Check sheet for the modelled part. Datum: model origin and axes. Units: mm. A direction names the side the tool comes from. Give positions to 0.01 mm unless a question says otherwise; leave off trailing zeros. Write each loop counter-clockwise with the first axis right and the second up, starting at its lowest first coordinate (ties: lowest second). Pieces come first, ordered by that corner, then holes. Notation, with made-up numbers: M 72,-26.75 L 130,-26.75 A13 ccw 130,-5.75 Z; hole C 59.5,-16.5 d10. An arc over 180 degrees is marked long. Write each question's results on one line, items separated by ' | '. Start each with the question number.
from build123d import *

# Parameters (mm, degrees)
SKETCH1_R           = 1.75
BOSS_EXTRUDE1_DEPTH = 10
BOSS_EXTRUDE2_DEPTH = 105
RIB1_REACH          = 140.024
SKETCH3_WALL_W      = 372.917163166
SKETCH3_WALL_H      = 6
FILLET1_R           = 2
FILLET2_R           = 4
SKETCH4_W           = 4
SKETCH4_H           = 13.56
CUT_EXTRUDE1_DEPTH  = 8


with BuildPart() as part:
    # Sketch1 → Boss-Extrude1 (new body)
    with BuildSketch(Plane.XY):
        Polygon((-45.99, 7.5), (-45.99, -7.5), (-17.99, -7.5), (-17.99, -53.64), (46, -53.64), (46, -38.64), (31.39, -38.64), (31.39, 7.5), align=None)
        Circle(SKETCH1_R, mode=Mode.SUBTRACT)
        with Locations((25.39, 0)):
            Circle(SKETCH1_R, mode=Mode.SUBTRACT)
        with Locations((-39.99, 0)):
            Circle(SKETCH1_R, mode=Mode.SUBTRACT)
        with Locations((40, -46.14)):
            Circle(SKETCH1_R, mode=Mode.SUBTRACT)
    extrude(amount=BOSS_EXTRUDE1_DEPTH)

    # Sketch2 → Boss-Extrude2 (add)
    with BuildSketch(Plane.XY.offset(10)):
        Polygon((-13.3, -5), (-3.3, -5), (-3.3, -18.56), (-13.3, -18.56), (-13.3, -12.56), (-8.3, -12.56), (-8.3, -10), (-13.3, -10), align=None)
    extrude(amount=BOSS_EXTRUDE2_DEPTH)

    # Sketch3 wall → Rib1 (add, up to next)
    with BuildSketch(Plane(origin=(-8.3, -33.56, 55), x_dir=(0, 0.316227766017, 0.948683298051), z_dir=(0, -0.948683298051, 0.316227766017)), mode=Mode.PRIVATE) as rib1_sk1:
        Rectangle(SKETCH3_WALL_W, SKETCH3_WALL_H)
    rib1_tool1 = extrude(rib1_sk1.sketch, amount=-RIB1_REACH, mode=Mode.PRIVATE) - part.part
    add(rib1_tool1.solids().sort_by_distance((-8.3, -33.56, 55))[0])

    # Fillet1
    fillet1_edges = [part.edges().sort_by_distance(p)[0] for p in [
        (-13.3, -7.5, 10),
        (-13.3, -15.56, 10),
        (-12.3, -18.56, 10),
        (-11.3, -33.56, 10),
        (-3.3, -11.78, 10),
        (-4.3, -18.56, 10),
        (-5.3, -33.56, 10),
    ]]
    fillet(fillet1_edges, radius=FILLET1_R)

    # Fillet2
    fillet2_edges = [part.edges().sort_by_distance(p)[0] for p in [
        (31.39, -38.64, 5),
        (-17.99, -53.64, 5),
        (-17.99, -7.5, 5),
    ]]
    fillet(fillet2_edges, radius=FILLET2_R)

    # Sketch4 → Cut-Extrude1 (cut)
    with BuildSketch(Plane.XY.offset(115)):
        with Locations((-8.3, -11.78)):
            Rectangle(SKETCH4_W, SKETCH4_H)
    extrude(amount=-CUT_EXTRUDE1_DEPTH, mode=Mode.SUBTRACT)


solid = part.part
Q1. Release check for a two-part mould opening along X. For faces 1 (the face through (-3.3, -12, 63)), 2 (the face through (-6.3, -12, 111)), 3 (the face through (-11, -10, 62)) record: pulls with the +X half, pulls with the -X half, needs draft (parallel to the pull), parting line crosses it, or undercut.
Q2. Scan lines: L1, parallel to Y at x = -39.99, z = 6.5; L2, parallel to Y at x = 40, z = 6.25; L3, parallel to X at y = -46, z = 7. Record each from-to range of solid material in increasing order.
Q3. Section check B-B on y = 0. Record the boundary of the cut face in (x, z).
Q4. Section check A-A on x = 40. Record the boundary of the cut face in (y, z).
Q5. Tool access check on faces 4 (the face through (31.39, -14, 5)), 5 (the face through (-8, -5, 62)), 6 (the face through (-11.3, -30, 43)), 7 (the face through (-8, -12, 107)), 8 (the face through (-17.99, -30, 5)). Record the directions out of +Z, -Z, +X, -X, +Y, -Y that give a thin tool (end or side, any length) a straight path to the whole face; none if there is none.
Q6. Depth check by flat-ended pin: pin 1 Ø12 at (x, z) = (11.5, 14.5) entering from -Y; pin 2 Ø3 at (x, y) = (0, 0) entering from -Z; pin 3 Ø1.5 at (x, z) = (-11, 24.5) entering from +Y; pin 4 Ø2.5 at (y, z) = (-7.5, 109) entering from +X. Enter the tip coordinate at first touch or a pass-through.
Q7. Section check D-D on x = 25.39. Record the boundary of the cut face in (y, z).
Q8. Section check C-C on z = 104.5. Record the boundary of the cut face in (x, y).
Check result:
1) face 1: pulls with the +X half | face 2: undercut | face 3: needs draft
2) L1: -7.5 to -1.75, 1.75 to 7.5 | L2: -53.64 to -47.89, -44.39 to -38.64 | L3: -17.99 to 38.26, 41.74 to 46
3) outline: M -45.99,0 L -41.74,0 L -41.74,10 L -45.99,10 Z; M -38.24,0 L -1.75,0 L -1.75,10 L -38.24,10 Z; M 1.75,0 L 23.64,0 L 23.64,10 L 1.75,10 Z; M 27.14,0 L 31.39,0 L 31.39,10 L 27.14,10 Z
4) outline: M -53.64,0 L -47.89,0 L -47.89,10 L -53.64,10 Z; M -44.39,0 L -38.64,0 L -38.64,10 L -44.39,10 Z
5) face 4: +Z, -Z, +X, +Y | face 5: +Z, +X, -X, +Y | face 6: +Z, -X, -Y | face 7: +Z, +Y, -Y | face 8: +Z, -Z, -X, -Y
6) pin 1: y = -53.64 | pin 2: through | pin 3: y = -5 | pin 4: x = -3.3
7) outline: M -53.64,0 L -1.75,0 L -1.75,10 L -53.64,10 Z; M 1.75,0 L 7.5,0 L 7.5,10 L 1.75,10 Z
8) outline: M -13.3,-18.56 L -3.3,-18.56 L -3.3,-5 L -13.3,-5 L -13.3,-10 L -8.3,-10 L -8.3,-12.56 L -13.3,-12.56 Z
